from build123d import *

# Parameters (mm, degrees)
SKETCH1_W                = 164.1
SKETCH1_H                = 174.745
BOSS_EXTRUDE1_DEPTH      = 1.5875
FILLET1_R                = 1
SKETCH2_R                = 1.4732
CUT_EXTRUDE1_DEPTH       = 10
HEAT_STRAP_CONNECTIONS_R = 1.4732
CUT_EXTRUDE2_DEPTH       = 241.065605994


with BuildPart() as part:
    # Sketch1 → Boss-Extrude1 (new body)
    with BuildSketch(Plane.XY):
        with Locations((82.55, -87.3725)):
            Rectangle(SKETCH1_W, SKETCH1_H)
        with BuildLine():
            Line((82.55, -5.4375), (80.434372699, -5.4375))
            ThreePointArc((80.434372699, -5.4375), (75.6625, -3.85), (80.434372699, -2.2625))
            Line((80.434372699, -2.2625), (82.55, -2.2625))
            ThreePointArc((82.55, -2.2625), (84.1375, -3.85), (82.55, -5.4375))
        make_face(mode=Mode.SUBTRACT)
        with BuildLine():
            Line((16.934372699, -168.395), (19.05, -168.395))
            ThreePointArc((19.05, -168.395), (20.6375, -169.9825), (19.05, -171.57))
            Line((19.05, -171.57), (16.934372699, -171.57))
            ThreePointArc((16.934372699, -171.57), (12.1625, -169.9825), (16.934372699, -168.395))
        make_face(mode=Mode.SUBTRACT)
        with BuildLine():
            Line((7.409372699, -151.9325), (9.525, -151.9325))
            ThreePointArc((9.525, -151.9325), (11.1125, -153.52), (9.525, -155.1075))
            Line((9.525, -155.1075), (7.409372699, -155.1075))
            ThreePointArc((7.409372699, -155.1075), (2.6375, -153.52), (7.409372699, -151.9325))
        make_face(mode=Mode.SUBTRACT)
        with BuildLine():
            Line((42.334372699, -168.395), (44.45, -168.395))
            ThreePointArc((44.45, -168.395), (46.0375, -169.9825), (44.45, -171.57))
            Line((44.45, -171.57), (42.334372699, -171.57))
            ThreePointArc((42.334372699, -171.57), (37.5625, -169.9825), (42.334372699, -168.395))
        make_face(mode=Mode.SUBTRACT)
        with BuildLine():
            Line((67.734372699, -168.395), (69.85, -168.395))
            ThreePointArc((69.85, -168.395), (71.4375, -169.9825), (69.85, -171.57))
            Line((69.85, -171.57), (67.734372699, -171.57))
            ThreePointArc((67.734372699, -171.57), (62.9625, -169.9825), (67.734372699, -168.395))
        make_face(mode=Mode.SUBTRACT)
        with BuildLine():
            Line((7.409372699, -126.5325), (9.525, -126.5325))
            ThreePointArc((9.525, -126.5325), (11.1125, -128.12), (9.525, -129.7075))
            Line((9.525, -129.7075), (7.409372699, -129.7075))
            ThreePointArc((7.409372699, -129.7075), (2.6375, -128.12), (7.409372699, -126.5325))
        make_face(mode=Mode.SUBTRACT)
        with BuildLine():
            Line((7.409372699, -101.1325), (9.525, -101.1325))
            ThreePointArc((9.525, -101.1325), (11.1125, -102.72), (9.525, -104.3075))
            Line((9.525, -104.3075), (7.409372699, -104.3075))
            ThreePointArc((7.409372699, -104.3075), (2.6375, -102.72), (7.409372699, -101.1325))
        make_face(mode=Mode.SUBTRACT)
        with BuildLine():
            Line((7.409372699, -75.7325), (9.525, -75.7325))
            ThreePointArc((9.525, -75.7325), (11.1125, -77.32), (9.525, -78.9075))
            Line((9.525, -78.9075), (7.409372699, -78.9075))
            ThreePointArc((7.409372699, -78.9075), (2.6375, -77.32), (7.409372699, -75.7325))
        make_face(mode=Mode.SUBTRACT)
        with BuildLine():
            Line((7.409372699, -50.3325), (9.525, -50.3325))
            ThreePointArc((9.525, -50.3325), (11.1125, -51.92), (9.525, -53.5075))
            Line((9.525, -53.5075), (7.409372699, -53.5075))
            ThreePointArc((7.409372699, -53.5075), (2.6375, -51.92), (7.409372699, -50.3325))
        make_face(mode=Mode.SUBTRACT)
        with BuildLine():
            Line((7.409372699, -24.9325), (9.525, -24.9325))
            ThreePointArc((9.525, -24.9325), (11.1125, -26.52), (9.525, -28.1075))
            Line((9.525, -28.1075), (7.409372699, -28.1075))
            ThreePointArc((7.409372699, -28.1075), (2.6375, -26.52), (7.409372699, -24.9325))
        make_face(mode=Mode.SUBTRACT)
        with BuildLine():
            Line((7.409372699, -8.1), (9.525, -8.1))
            ThreePointArc((9.525, -8.1), (11.1125, -9.6875), (9.525, -11.275))
            Line((9.525, -11.275), (7.409372699, -11.275))
            ThreePointArc((7.409372699, -11.275), (2.6375, -9.6875), (7.409372699, -8.1))
        make_face(mode=Mode.SUBTRACT)
        with BuildLine():
            Line((29.634372699, -2.2625), (31.75, -2.2625))
            ThreePointArc((31.75, -2.2625), (33.3375, -3.85), (31.75, -5.4375))
            Line((31.75, -5.4375), (29.634372699, -5.4375))
            ThreePointArc((29.634372699, -5.4375), (24.8625, -3.85), (29.634372699, -2.2625))
        make_face(mode=Mode.SUBTRACT)
        with BuildLine():
            Line((55.034372699, -2.2625), (57.15, -2.2625))
            ThreePointArc((57.15, -2.2625), (58.7375, -3.85), (57.15, -5.4375))
            Line((57.15, -5.4375), (55.034372699, -5.4375))
            ThreePointArc((55.034372699, -5.4375), (50.2625, -3.85), (55.034372699, -2.2625))
        make_face(mode=Mode.SUBTRACT)
        with BuildLine():
            ThreePointArc((161.925, -8.1), (163.5125, -9.6875), (161.925, -11.275))
            Line((161.925, -11.275), (159.809372699, -11.275))
            ThreePointArc((159.809372699, -11.275), (155.0375, -9.6875), (159.809372699, -8.1))
            Line((159.809372699, -8.1), (161.925, -8.1))
        make_face(mode=Mode.SUBTRACT)
        with BuildLine():
            Line((93.134372699, -168.395), (95.25, -168.395))
            ThreePointArc((95.25, -168.395), (96.8375, -169.9825), (95.25, -171.57))
            Line((95.25, -171.57), (93.134372699, -171.57))
            ThreePointArc((93.134372699, -171.57), (88.3625, -169.9825), (93.134372699, -168.395))
        make_face(mode=Mode.SUBTRACT)
        with BuildLine():
            Line((118.534372699, -168.395), (120.65, -168.395))
            ThreePointArc((120.65, -168.395), (122.2375, -169.9825), (120.65, -171.57))
            Line((120.65, -171.57), (118.534372699, -171.57))
            ThreePointArc((118.534372699, -171.57), (113.7625, -169.9825), (118.534372699, -168.395))
        make_face(mode=Mode.SUBTRACT)
        with BuildLine():
            Line((143.934372699, -168.395), (146.05, -168.395))
            ThreePointArc((146.05, -168.395), (147.6375, -169.9825), (146.05, -171.57))
            Line((146.05, -171.57), (143.934372699, -171.57))
            ThreePointArc((143.934372699, -171.57), (139.1625, -169.9825), (143.934372699, -168.395))
        make_face(mode=Mode.SUBTRACT)
        with BuildLine():
            Line((159.809372699, -151.9325), (161.925, -151.9325))
            ThreePointArc((161.925, -151.9325), (163.5125, -153.52), (161.925, -155.1075))
            Line((161.925, -155.1075), (159.809372699, -155.1075))
            ThreePointArc((159.809372699, -155.1075), (155.0375, -153.52), (159.809372699, -151.9325))
        make_face(mode=Mode.SUBTRACT)
        with BuildLine():
            Line((159.809372699, -126.5325), (161.925, -126.5325))
            ThreePointArc((161.925, -126.5325), (163.5125, -128.12), (161.925, -129.7075))
            Line((161.925, -129.7075), (159.809372699, -129.7075))
            ThreePointArc((159.809372699, -129.7075), (155.0375, -128.12), (159.809372699, -126.5325))
        make_face(mode=Mode.SUBTRACT)
        with BuildLine():
            Line((159.809372699, -101.1325), (161.925, -101.1325))
            ThreePointArc((161.925, -101.1325), (163.5125, -102.72), (161.925, -104.3075))
            Line((161.925, -104.3075), (159.809372699, -104.3075))
            ThreePointArc((159.809372699, -104.3075), (155.0375, -102.72), (159.809372699, -101.1325))
        make_face(mode=Mode.SUBTRACT)
        with BuildLine():
            Line((159.809372699, -75.7325), (161.925, -75.7325))
            ThreePointArc((161.925, -75.7325), (163.5125, -77.32), (161.925, -78.9075))
            Line((161.925, -78.9075), (159.809372699, -78.9075))
            ThreePointArc((159.809372699, -78.9075), (155.0375, -77.32), (159.809372699, -75.7325))
        make_face(mode=Mode.SUBTRACT)
        with BuildLine():
            Line((159.809372699, -50.3325), (161.925, -50.3325))
            ThreePointArc((161.925, -50.3325), (163.5125, -51.92), (161.925, -53.5075))
            Line((161.925, -53.5075), (159.809372699, -53.5075))
            ThreePointArc((159.809372699, -53.5075), (155.0375, -51.92), (159.809372699, -50.3325))
        make_face(mode=Mode.SUBTRACT)
        with BuildLine():
            Line((105.834372699, -2.2625), (107.95, -2.2625))
            ThreePointArc((107.95, -2.2625), (109.5375, -3.85), (107.95, -5.4375))
            Line((107.95, -5.4375), (105.834372699, -5.4375))
            ThreePointArc((105.834372699, -5.4375), (101.0625, -3.85), (105.834372699, -2.2625))
        make_face(mode=Mode.SUBTRACT)
        with BuildLine():
            Line((159.809372699, -24.9325), (161.925, -24.9325))
            ThreePointArc((161.925, -24.9325), (163.5125, -26.52), (161.925, -28.1075))
            Line((161.925, -28.1075), (159.809372699, -28.1075))
            ThreePointArc((159.809372699, -28.1075), (155.0375, -26.52), (159.809372699, -24.9325))
        make_face(mode=Mode.SUBTRACT)
        with BuildLine():
            Line((131.234372699, -2.2625), (133.35, -2.2625))
            ThreePointArc((133.35, -2.2625), (134.9375, -3.85), (133.35, -5.4375))
            Line((133.35, -5.4375), (131.234372699, -5.4375))
            ThreePointArc((131.234372699, -5.4375), (126.4625, -3.85), (131.234372699, -2.2625))
        make_face(mode=Mode.SUBTRACT)
    extrude(amount=BOSS_EXTRUDE1_DEPTH)

    # Fillet1
    fillet1_edges = [part.edges().sort_by_distance(p)[0] for p in [
        (164.6, -174.745, 0.79375),
        (0.5, -174.745, 0.79375),
        (0.5, 0, 0.79375),
        (164.6, 0, 0.79375),
    ]]
    fillet(fillet1_edges, radius=FILLET1_R)

    # Sketch2 → Cut-Extrude1 (cut)
    with BuildSketch(Plane.XY.offset(1.5875)):
        Polygon((117.55, -86.8725), (47.55, -86.8725), (47.55, -126.8725), (47.55, -131.8725), (117.55, -131.8725), (117.55, -126.8725), align=None)
        with Locations((110.05, -76.8725)):
            Circle(SKETCH2_R)
        with Locations((37.55, -94.3725)):
            Circle(SKETCH2_R)
        with Locations((37.55, -124.3725)):
            Circle(SKETCH2_R)
        with Locations((110.05, -141.8725)):
            Circle(SKETCH2_R)
        with Locations((55.05, -141.8725)):
            Circle(SKETCH2_R)
        with Locations((55.05, -76.8725)):
            Circle(SKETCH2_R)
        with Locations((127.55, -94.3725)):
            Circle(SKETCH2_R)
        with Locations((127.55, -124.3725)):
            Circle(SKETCH2_R)
    extrude(amount=-CUT_EXTRUDE1_DEPTH, mode=Mode.SUBTRACT)

    # Heat Strap Connections → Cut-Extrude2 (cut, through all)
    with BuildSketch(Plane.XY.offset(1.5875)):
        with Locations((38.1, -48.175)):
            Circle(HEAT_STRAP_CONNECTIONS_R)
        with Locations((50.8, -48.175)):
            Circle(HEAT_STRAP_CONNECTIONS_R)
        with Locations((63.5, -48.175)):
            Circle(HEAT_STRAP_CONNECTIONS_R)
        with Locations((76.2, -48.175)):
            Circle(HEAT_STRAP_CONNECTIONS_R)
        with Locations((88.9, -48.175)):
            Circle(HEAT_STRAP_CONNECTIONS_R)
        with Locations((101.6, -48.175)):
            Circle(HEAT_STRAP_CONNECTIONS_R)
        with Locations((114.3, -48.175)):
            Circle(HEAT_STRAP_CONNECTIONS_R)
        with Locations((127, -48.175)):
            Circle(HEAT_STRAP_CONNECTIONS_R)
        with Locations((23.5, -149.3975)):
            Circle(HEAT_STRAP_CONNECTIONS_R)
        with Locations((141.6, -149.3975)):
            Circle(HEAT_STRAP_CONNECTIONS_R)
        with Locations((36.2, -149.3975)):
            Circle(HEAT_STRAP_CONNECTIONS_R)
        with Locations((128.9, -149.3975)):
            Circle(HEAT_STRAP_CONNECTIONS_R)
    extrude(amount=-CUT_EXTRUDE2_DEPTH, mode=Mode.SUBTRACT)


solid = part.part
Work out the finished part from the listing and answer in its coordinate system (mm). Round coordinates to 2 decimals unless told otherwise and drop trailing zeros. Write each loop counter-clockwise with the first axis right and the second up, starting at its lowest first coordinate (ties: lowest second). Pieces come first, ordered by that corner, then holes. Notation, with made-up numbers: (61.5, 68.5) - (102.5, 68.5) arc R20 ccw to (102.5, 106.5) - close; hole circle Ø5 at (20, 0). An arc over 180 degrees is marked (long way). Answer in a Markdown table with one row per item. Add a question column.
1. Given pin 1 (4 mm diameter, centred on x = 141.81, y = -169.98, fed in from -Z); pin 2 (7 mm diameter, centred on x = 5.29, y = -128.12, fed in from +Z), each flat-ended and moving along its own axis, determine where each tip first touches the part or whether it passes through.
2. The mould has two halves that part along Y. Classify faces 1 (the cylindrical face through (62.964, -170.075, 0.783)), 2 (the flat face through (81, -86, 0)), 3 (the cylindrical face through (139.164, -170.075, 0.783)): +Y half, -Y half, draft (parallel to the pull), parting line (faces both ways), or undercut.
3. A cutting plane is placed at A-A, the plane y = -113. Determine the outline of the cut face in (x, z), and give its area (3 significant figures).
4. Find the intervals of material crossed by line 1 along Y through (x, z) = (63.5, 1.4) (1 decimal); line 2 along Y through (x, z) = (82.5, 1.1) (1 decimal); line 3 along Y through (x, z) = (110.05, 0.95) (1 decimal), in increasing order. Write a range as from..to.
5. A cutting plane is placed at B-B, the plane z = 0.5. Count the separate pieces of the cut face and the enclosed holes in it, and give its area (3 significant figures).
Worked out:
| question | item | result |
|---|---|---|
| 1 | pin 1 | through |
| 1 | pin 2 | z = 1.59 |
| 2 | face 1 | undercut |
| 2 | face 2 | draft |
| 2 | face 3 | undercut |
| 3 | outline | (0.5, 0) - (47.55, 0) - (47.55, 1.59) - (0.5, 1.59) - close; (117.55, 0) - (164.6, 0) - (164.6, 1.59) - (117.55, 1.59) - close |
| 3 | area | 149 mm^2 |
| 4 | line 1 | -174.7..-171.6, -168.4..-131.9, -86.9..-49.6, -46.7..0 |
| 4 | line 2 | -174.7..-131.9, -86.9..-5.4, -2.3..0 |
| 4 | line 3 | -174.7..-143.3, -140.4..-131.9, -86.9..-78.3, -75.4..0 |
| 5 | separate pieces | 1 |
| 5 | enclosed holes | 46 |
| 5 | area | 24,600 mm^2 |
